from build123d import *

# Parameters (mm, degrees)
F0_W          = 130
F0_H          = 13
F1_DEPTH      = 25
F2_R          = 4
F3_DEPTH      = 25
F3_FACE_R     = 4
F4_DEPTH      = 99.4
F5_R          = 5
F6_R          = 4
F7_DEPTH      = 13
F7_DEPTH_BACK = 25


with BuildPart() as f1:
    # F0 (on Top) → F1 (new body)
    with BuildSketch(Plane.XY):
        with Locations((-7.093077, -51.712683)):
            Rectangle(F0_W, F0_H)
    extrude(amount=F1_DEPTH)

    # F2 (on face) → F3 (join)
    with BuildSketch(Plane(origin=(0, -45.212683, 0), x_dir=(-1, 0, 0), z_dir=(0, 1, 0))):
        with Locations((-39.799914, 11.472573)):
            Circle(F2_R)
        with Locations((56.796312, 11.472573)):
            Circle(F2_R)
    extrude(amount=F3_DEPTH)

    # F3_face (on face) → F4 (cut)
    with BuildSketch(Plane(origin=(39.799914, -20.212683, 11.472573), x_dir=(-1, 0, 0), z_dir=(0, 1, 0))):
        Circle(F3_FACE_R)
        with Locations((96.596226, 0)):
            Circle(F3_FACE_R)
    extrude(amount=-F4_DEPTH, mode=Mode.SUBTRACT)

    # F5
    f5_edges = [f1.edges().sort_by_distance(p)[0] for p in [
        (57.906923, -51.712683, 25),
        (57.906923, -51.712683, 0),
        (-7.093077, -58.212683, 25),
        (-7.093077, -45.212683, 25),
    ]]
    fillet(f5_edges, radius=F5_R)

    # F6 (on face) → F7 (join, two sides)
    with BuildSketch(Plane.XZ.offset(58.212683)) as f7_sk:
        with Locations((-56.796312, 11.472573)):
            Circle(F6_R)
        with Locations((39.799914, 11.472573)):
            Circle(F6_R)
    extrude(amount=F7_DEPTH)
    extrude(f7_sk.sketch, amount=-F7_DEPTH_BACK)


solid = f1.part
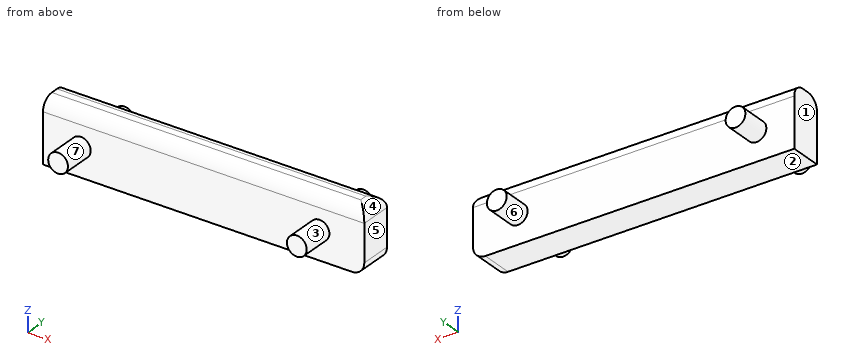
Work out the finished part from the listing and answer in its coordinate system (mm). Face numbers are marked on the shaded views. A direction names the side the tool comes from. Give positions to 0.01 mm unless a question says otherwise; leave off trailing zeros. Write each loop counter-clockwise with the first axis right and the second up, starting at its lowest first coordinate (ties: lowest second). Pieces come first, ordered by that corner, then holes. Notation, with made-up numbers: M 11.5,45.25 L 68.5,45.25 A6 ccw 68.5,52.25 Z; hole C -33.5,-37 d7. An arc over 180 degrees is marked long. Answer as CSV lines item,"result".
Q1. A cutting plane is placed at A-A on x = -20.5. Write down the section's boundary in (y, z), plus the area to 3 significant figures.
A:
outline,"M -58.21,0 L -45.21,0 L -45.21,20 A5 ccw -50.21,25 L -53.21,25 A5 ccw -58.21,20 Z"
area,"314 mm²"
Q2. A cutting plane is placed at B-B on y = -48.5. Write down the section's boundary in (x, z).
A:
outline,"M -72.09,0 L 52.91,0 A5 ccw 57.91,5 L 57.91,20 A5 ccw 54.62,24.7 L -72.09,24.7 Z"
Q3. Find the intervals of material crossed by probe 1 along X at (y, z) = (-67.5, 11.75); probe 2 along Y at (x, z) = (-17, 3); probe 3 along X at (y, z) = (-59, 8.75), in increasing order. Write a range as [from, to].
A:
probe 1,"x = [-60.79, -52.81], [35.81, 43.79]"
probe 2,"y = [-58.21, -45.21]"
probe 3,"x = [-59.73, -53.87], [36.87, 42.73]"
Q4. A cutting plane is placed at C-C on z = 18.75. Write down the section's boundary in (x, y), plus the area to 3 significant figures.
A:
outline,"M -72.09,-58.21 L 57.91,-58.21 L 57.91,-45.21 L -72.09,-45.21 Z"
area,"1,690 mm²"
Q5. A tool of negligible diameter and unlimited length cuts with its end or side. For the marked faces 5, 6 and 7, from which of +Z, -Z, +X, -X, +Y, -Y can it reach the whole face along a straight path? Write none if from no direction.
A:
face 5,"+Z, -Z, +X, +Y, -Y"
face 6,"+Y"
face 7,"-Y"
Q6. Given P1, Ø6, axis at x = 34.5, y = -37.5, coming from the -Z side; P2, Ø1.5, axis at x = -19, z = 3.5, coming from the -Y side; P3, Ø4, axis at x = -15.5, z = 22, coming from the +Y side, each flat-ended and moving along its own axis, determine where each tip first touches the part or whether it passes through.
A:
P1,"stops at z = 8.2"
P2,"stops at y = -58.21"
P3,"stops at y = -45.21"
Q7. A cutting plane is placed at D-D on y = -37. Write down the section's boundary in (x, z), plus the area to 3 significant figures.
A:
outline,"C -56.8,11.47 d8; C 39.8,11.47 d8"
area,"101 mm²"
Q8. The mould has two halves that part along X. Classify the marked faces 1, 2, 3 and 4: +X half, -X half, draft (parallel to the pull), parting line (faces both ways), or undercut.
A:
face 1,"-X half"
face 2,"draft"
face 3,"undercut"
face 4,"+X half"
